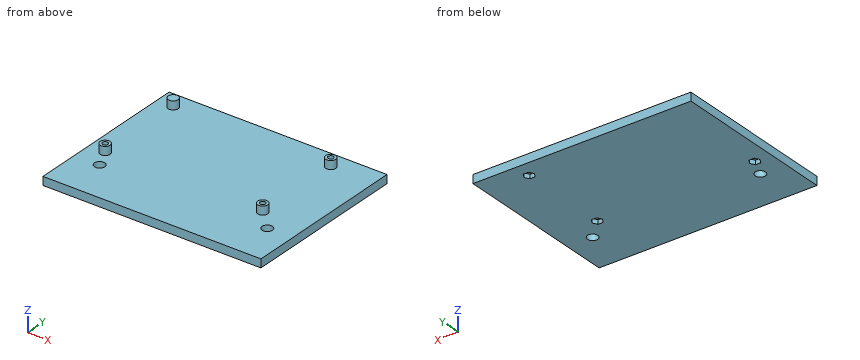
from build123d import *

# Parameters (mm, degrees)
SKETCH001_W     = 130
SKETCH001_H     = 100
PAD001_DEPTH    = 5
SKETCH002_R     = 3
PAD002_DEPTH    = 5
SKETCH003_R     = 1.6
POCKET_DEPTH    = 10
POCKET005_DEPTH = 2.5
SKETCH013_R     = 3.1
POCKET006_DEPTH = 5


with BuildPart() as part:
    # Sketch001 → Pad001 (new body)
    with BuildSketch(Plane.XY):
        with Locations((65, 50)):
            Rectangle(SKETCH001_W, SKETCH001_H)
    extrude(amount=PAD001_DEPTH)

    # Sketch002 (on Face6 of Pad001) → Pad002 (join)
    with BuildSketch(Plane.XY.offset(5)):
        with Locations((10, 90)):
            Circle(SKETCH002_R)
        with Locations((10, 36)):
            Circle(SKETCH002_R)
        with Locations((104, 90)):
            Circle(SKETCH002_R)
        with Locations((104, 36)):
            Circle(SKETCH002_R)
    extrude(amount=PAD002_DEPTH)

    # Sketch003 (on Face4 of Pad002) → Pocket (cut)
    with BuildSketch(Plane(origin=(0, 0, 0), x_dir=(1, 0, 0), z_dir=(0, 0, -1))):
        with Locations((10, -36)):
            Circle(SKETCH003_R)
        with Locations((104, -36)):
            Circle(SKETCH003_R)
        with Locations((104, -90)):
            Circle(SKETCH003_R)
    extrude(amount=-POCKET_DEPTH, mode=Mode.SUBTRACT)

    # Sketch012 (on Face4 of Pocket) → Pocket005 (cut)
    with BuildSketch(Plane(origin=(0, 0, 0), x_dir=(1, 0, 0), z_dir=(0, 0, -1))):
        Polygon((107.1, -90), (105.55, -87.315321), (102.45, -87.315321), (100.9, -90), (102.45, -92.684679), (105.55, -92.684679), align=None)
        Polygon((13.1, -36), (11.55, -33.315321), (8.45, -33.315321), (6.9, -36), (8.45, -38.684679), (11.55, -38.684679), align=None)
        Polygon((107.1, -36), (105.55, -33.315321), (102.45, -33.315321), (100.9, -36), (102.45, -38.684679), (105.55, -38.684679), align=None)
    extrude(amount=-POCKET005_DEPTH, mode=Mode.SUBTRACT)

    # Sketch013 (on Face6 of Pad001) → Pocket006 (cut)
    with BuildSketch(Plane.XY.offset(5)):
        with Locations((115, 25)):
            Circle(SKETCH013_R)
        with Locations((15, 25)):
            Circle(SKETCH013_R)
    extrude(amount=-POCKET006_DEPTH, mode=Mode.SUBTRACT)


solid = part.part
Input: part model. Units: mm. Frame: model coordinates. Coordinates: 2 decimals unless noted, no trailing zeros. Loops run counter-clockwise (first coordinate to the right, second up) from the corner with the lowest first, then second, coordinate; pieces in that order, holes last.
Q1. Material intervals for line 1 (Y direction, x = 104, z = 7); line 2 (Y direction, x = 15, z = 1.6); line 3 (Y direction, x = 104, z = 3.5), sorted ascending.
Q2. Cut plane A-A (x = 10). Output: boundary loops of the cut face in (y, z), then the cut area to 3 significant figures.
Q3. Cut plane C-C (x = 104). Output: boundary loops of the cut face in (y, z).
Q4. Cut plane B-B (y = 25). Output: boundary loops of the cut face in (x, z).
Q5. Cut plane D-D (y = 62). Output: boundary loops of the cut face in (x, z), then the cut area to 3 significant figures.
Q6. Contact query for flat-ended pins moving along their axis: pin 1 (6 mm diameter, centred on x = 75, y = 89, fed in from +Z); pin 2 (5.5 mm diameter, centred on x = 115, y = 25, fed in from +Z); pin 3 (4 mm diameter, centred on x = 104, y = 90, fed in from -Z). Output: stop coordinate, or through.
Working result:
1. line 1: y = 33 to 34.4, 37.6 to 39, 87 to 88.4, 91.6 to 93
1. line 2: y = 0 to 21.9, 28.1 to 100
1. line 3: y = 0 to 34.4, 37.6 to 88.4, 91.6 to 100
2. outline: (0, 0) - (33.32, 0) - (33.32, 2.5) - (34.4, 2.5) - (34.4, 10) - (33, 10) - (33, 5) - (0, 5) - close; (37.6, 2.5) - (38.68, 2.5) - (38.68, 0) - (100, 0) - (100, 5) - (93, 5) - (93, 10) - (87, 10) - (87, 5) - (39, 5) - (39, 10) - (37.6, 10) - close
2. area: 523 mm2
3. outline: (0, 0) - (33.32, 0) - (33.32, 2.5) - (34.4, 2.5) - (34.4, 10) - (33, 10) - (33, 5) - (0, 5) - close; (37.6, 2.5) - (38.68, 2.5) - (38.68, 0) - (87.32, 0) - (87.32, 2.5) - (88.4, 2.5) - (88.4, 10) - (87, 10) - (87, 5) - (39, 5) - (39, 10) - (37.6, 10) - close; (91.6, 2.5) - (92.68, 2.5) - (92.68, 0) - (100, 0) - (100, 5) - (93, 5) - (93, 10) - (91.6, 10) - close
4. outline: (0, 0) - (11.9, 0) - (11.9, 5) - (0, 5) - close; (18.1, 0) - (111.9, 0) - (111.9, 5) - (18.1, 5) - close; (118.1, 0) - (130, 0) - (130, 5) - (118.1, 5) - close
5. outline: (0, 0) - (130, 0) - (130, 5) - (0, 5) - close
5. area: 650 mm2
6. pin 1: stops at z = 5
6. pin 2: passes through
6. pin 3: stops at z = 2.5
